```python
from build123d import *

# Parameters (mm, degrees)
F0_R     = 3.175
F1_DEPTH = 3.175


with BuildPart() as f1:
    # F0 (on Top) → F1 (new body)
    with BuildSketch(Plane.XY):
        with BuildLine():
            Line((43.77051, 9.500732), (0, 7.9375))
            ThreePointArc((0, 7.9375), (-7.9375, 0), (0, -7.9375))
            Line((0, -7.9375), (25.320855, -8.841816))
            ThreePointArc((25.320855, -8.841816), (31.19345, -11.634219), (33.181066, -17.825685))
            Line((33.181066, -17.825685), (28.712627, -63.5))
            Line((28.712627, -63.5), (34.925, -114.3))
            ThreePointArc((34.925, -114.3), (44.45, -123.825), (53.975, -114.3))
            Line((53.975, -114.3), (60.071, -63.5))
            Line((60.071, -63.5), (53.975, 0))
            ThreePointArc((53.975, 0), (51.185192, 6.735192), (44.45, 9.525))
            Line((44.45, 9.525), (43.77051, 9.500732))
        make_face()
        with Locations((44.45, -114.3)):
            Circle(F0_R, mode=Mode.SUBTRACT)
        with Locations((47.625, -100.0125)):
            Circle(F0_R, mode=Mode.SUBTRACT)
        with Locations((44.45, -63.5)):
            Circle(F0_R, mode=Mode.SUBTRACT)
        Circle(F0_R, mode=Mode.SUBTRACT)
        with Locations((44.45, 0)):
            Circle(F0_R, mode=Mode.SUBTRACT)
    extrude(amount=F1_DEPTH)


solid = f1.part
```
Source: CAD feature listing. Evaluate the final solid. Frame: model axes, mm. A direction names the side the tool comes from. Coordinates: 2 decimals unless noted, no trailing zeros. Loops run counter-clockwise (first coordinate to the right, second up) from the corner with the lowest first, then second, coordinate; pieces in that order, holes last. Notation, with made-up numbers: M 65.5,59 L 77.5,59 A22 ccw 77.5,87 Z; hole C -26.5,75 d10. An arc over 180 degrees is marked long. Use a Markdown table: item, result. Add a question column.
Q1. Section query B-B, the plane x = 52. Return loops of the section in (y, z) (3 decimals).
Q2. Section query C-C, the plane y = -43.5. Return loops of the section in (x, z) (3 decimals), and give its area (3 significant figures).
Q3. Access query for faces 5 (the cylindrical face through (31.13, -11.56, 1.57)), 6 (the flat face through (41, -41, 3.175)). Directions: +Z, -Z, +X, -X, +Y, -Y. A direction counts if a zero-diameter tool reaches every point of the face in a straight line with its end or side. Return the directions, or none.
Q4. First-contact query: pin 1 (12 mm diameter, centred on x = 20, y = -83.5, fed in from +Z); pin 2 (1 mm diameter, centred on x = -0.5, z = 1, fed in from +Y). Flat tips, straight axial feed; report the tip coordinate or a pass-through.
Q5. Material intervals for L1, parallel to Y at x = 42.5, z = 1.45; L2, parallel to X at y = -116.5, z = 2.7; L3, parallel to X at y = -66, z = 2.8, sorted ascending.
Q6. Draft query along X for faces 1 (the cylindrical face through (-0.69, -3.1, 1.57)), 2 (the flat face through (56.98, -89.26, 1.57)), 3 (the cylindrical face through (44.241, -123.823, 1.565)), 4 (the cylindrical face through (43.76, -117.4, 1.57)). Return one class per face: pulls with the +X half, pulls with the -X half, needs draft (parallel to the pull), parting line crosses it, or undercut.
Q7. Section query A-A, the plane z = 1.85. State how many separate pieces and enclosed holes the cut face has, and give its area (3 significant figures).
Result:
| question | item | result |
|---|---|---|
| 1 | outline | M -120.107,0 L 5.807,0 L 5.807,3.175 L -120.107,3.175 Z |
| 2 | outline | M 30.669,0 L 58.151,0 L 58.151,3.175 L 30.669,3.175 Z |
| 2 | area | 87.3 mm2 |
| 3 | face 5 | +Z, -Z, -X |
| 3 | face 6 | +Z, +X, -X, +Y, -Y |
| 4 | pin 1 | passes through |
| 4 | pin 2 | stops at y = 7.94 |
| 5 | L1 | y = -123.62 to -116.81, -111.79 to -66.01, -60.99 to -2.51, 2.51 to 9.46 |
| 5 | L2 | x = 35.18 to 42.16, 46.74 to 53.72 |
| 5 | L3 | x = 29.02 to 42.49, 46.41 to 59.77 |
| 6 | face 1 | undercut |
| 6 | face 2 | pulls with the +X half |
| 6 | face 3 | parting line crosses it |
| 6 | face 4 | undercut |
| 7 | separate pieces | 1 |
| 7 | enclosed holes | 5 |
| 7 | area | 3,730 mm2 |
